from build123d import *

# Parameters (mm, degrees)
F0_W     = 26
F0_H     = 26
F0_R     = 1
F1_DEPTH = 1
F2_W     = 11
F2_H     = 5
F3_DEPTH = 6
F4_W     = 8
F4_H     = 8
F5_DEPTH = 2
F6_R     = 3
F7_DEPTH = 5
F8_R     = 5
F9_DEPTH = 3


with BuildPart() as f1:
    # F0 (on Front) → F1 (new body)
    with BuildSketch(Plane.XZ):
        Rectangle(F0_W, F0_H)
        with Locations((-11, -11)):
            Circle(F0_R, mode=Mode.SUBTRACT)
        with Locations((11, -11)):
            Circle(F0_R, mode=Mode.SUBTRACT)
        with Locations((-10, 0)):
            Circle(F0_R, mode=Mode.SUBTRACT)
        with Locations((-11, 11)):
            Circle(F0_R, mode=Mode.SUBTRACT)
        with Locations((10, 0)):
            Circle(F0_R, mode=Mode.SUBTRACT)
        with Locations((11, 11)):
            Circle(F0_R, mode=Mode.SUBTRACT)
    extrude(amount=F1_DEPTH)

    # F2 (on face) → F3 (join)
    with BuildSketch(Plane(origin=(0, 0, 0), x_dir=(-1, 0, 0), z_dir=(0, 1, 0))):
        with Locations((-3.5, -12)):
            Rectangle(F2_W, F2_H)
    extrude(amount=F3_DEPTH)

    # F4 (on face) → F5 (join)
    with BuildSketch(Plane.XZ.offset(1)):
        Rectangle(F4_W, F4_H)
    extrude(amount=F5_DEPTH)

    # F6 (on face) → F7 (join)
    with BuildSketch(Plane.XZ.offset(3)):
        Circle(F6_R)
    extrude(amount=F7_DEPTH)

    # F8 (on face) → F9 (join)
    with BuildSketch(Plane.XZ.offset(8)):
        Circle(F8_R)
    extrude(amount=F9_DEPTH)


solid = f1.part
Design review of the part built by this model. Coordinates are the model's own, in mm. A direction names the side the tool comes from. Coordinates: 2 decimals unless noted, no trailing zeros. Order: outer loops, then holes, each group sorted by start corner. A loop starts at its lowest first (then second) coordinate and runs counter-clockwise, first axis right, second up. Notation, with made-up numbers: (11, 17) -> (18, 17) arc R8 ccw to (18, 29) -> close; hole circle Ø9 at (17, -37.5). An arc over 180 degrees is marked (long way). Use one line per item in the form item = value. Start each with the question number.
(1) Insertion check: pin 1 (2.5 mm diameter, centred on y = 3.5, z = -11, fed in from +X); pin 2 (3 mm diameter, centred on y = 0.5, z = -3.5, fed in from +X); pin 3 (6 mm diameter, centred on x = 9, z = -6.5, fed in from -Y); pin 4 (2 mm diameter, centred on x = -1, y = -1.5, fed in from -Z). Each pin has a flat end and moves straight along its axis. Give the tip position at first contact, or say it passes through.
(2) Add section C-C on z = -11. State the section outline as (x, y) points, plus the area to 3 significant figures.
(3) Add section D-D on y = -6. State the section outline as (x, z) points.
(4) Add section B-B on x = 7.5. State the section outline as (y, z) points, plus the area to 3 significant figures.
(5) Add section A-A on z = 11. State the section outline as (x, y) points.
(6) For probe 1 along Y at (x, z) = (-2.75, 2); probe 2 along Y at (x, z) = (-5, 9.25); probe 3 along Z at (x, y) = (6.25, 3.25), list the stretches that pass through material, from the lowest coordinate up.
(7) For faces 1 (the flat face through (4, 0, -14)), 2 (the flat face through (2, -3, 3)), 3 (the flat face through (4, -2, 0)), list the 3-axis set-ups (+Z, -Z, +X, -X, +Y, -Y) from which the entire face can be reached by the end or side of a thin tool; tool diameter is ignored.
(8) The part is to be moulded in two halves that separate along X. For faces 4 (the cylindrical face through (-3, -5, 0)), 5 (the cylindrical face through (-11.8, -0.5, 10.4)), 6 (the flat face through (0, -11, 0)), 7 (the cylindrical face through (9.2, -0.5, -0.6)), say which applies: +X half, -X half, draft (parallel to the pull), parting line (faces both ways), or undercut.
Answer block:
q1.pin_1 = 9
q1.pin_2 = 13
q1.pin_3 = -1
q1.pin_4 = -13
q2.outline = (-13, -1) -> (-12, -1) -> (-12, 0) -> (-13, 0) -> close; (-10, -1) -> (10, -1) -> (10, 0) -> (9, 0) -> (9, 6) -> (-2, 6) -> (-2, 0) -> (-10, 0) -> close; (12, -1) -> (13, -1) -> (13, 0) -> (12, 0) -> close
q2.area = 88.0 mm²
q3.outline = circle Ø6 at (0, 0)
q4.outline = (-1, -13) -> (0, -13) -> (0, -14.5) -> (6, -14.5) -> (6, -9.5) -> (0, -9.5) -> (0, 13) -> (-1, 13) -> close
q4.area = 56.0 mm²
q5.outline = (-13, -1) -> (-12, -1) -> (-12, 0) -> (-13, 0) -> close; (-10, -1) -> (10, -1) -> (10, 0) -> (-10, 0) -> close; (12, -1) -> (13, -1) -> (13, 0) -> (12, 0) -> close
q6.probe_1 = -11 to -8, -3 to 0
q6.probe_2 = -1 to 0
q6.probe_3 = -14.5 to -9.5
q7.face_1 = -Z, +X, -X, -Y
q7.face_2 = none
q7.face_3 = +Z, -Z, +X
q8.face_4 = parting line
q8.face_5 = undercut
q8.face_6 = draft
q8.face_7 = undercut
